Geometry: final body of the model. Coordinates: model frame, mm. Coordinates: 2 decimals unless noted, no trailing zeros. Order: outer loops, then holes, each group sorted by start corner. A loop starts at its lowest first (then second) coordinate and runs counter-clockwise, first axis right, second up. Notation, with made-up numbers: (50, 26.5) - (59, 26.5) arc R8 ccw to (59, 32.5) - close; hole circle Ø1 at (26, 79.25). An arc over 180 degrees is marked (long way). Use a Markdown table: item, result. Add a question column.
```python
from build123d import *

# Parameters (mm, degrees)
F0_W     = 276
F0_H     = 126
F1_DEPTH = 12
F2_R     = 5
F4_W     = 400
F4_H     = 300
F5_DEPTH = 10
F6_R     = 5


with BuildPart() as f1:
    # F0 (on Top) → F1 (new body)
    with BuildSketch(Plane.XY):
        Rectangle(F0_W, F0_H)
    extrude(amount=F1_DEPTH)

    # F2
    f2_edges = [f1.edges().sort_by_distance(p)[0] for p in [
        (0, -63, 12),
        (-138, 0, 12),
        (138, 0, 12),
        (0, 63, 12),
    ]]
    fillet(f2_edges, radius=F2_R)


with BuildPart() as f5:
    # F4 (on Top) → F5 (new body)
    with BuildSketch(Plane.XY):
        Rectangle(F4_W, F4_H)
    extrude(amount=F5_DEPTH)

    # F6
    f6_edges = [f5.edges().sort_by_distance(p)[0] for p in [
        (0, -150, 10),
        (-200, 0, 10),
        (200, 0, 10),
        (0, 150, 10),
    ]]
    fillet(f6_edges, radius=F6_R)


solid = f5.part
```
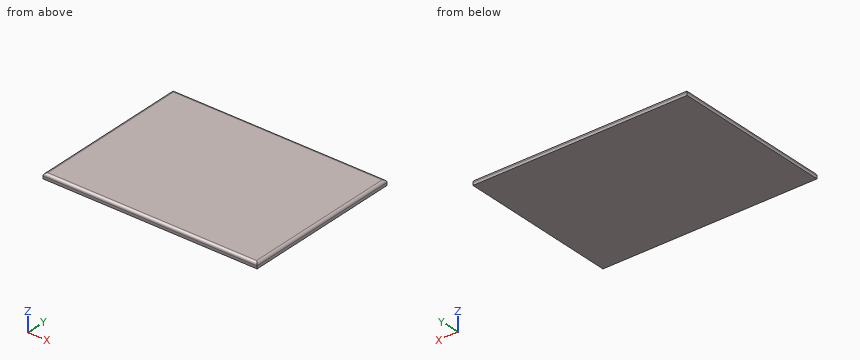
1) First-contact query: pin 1 (5 mm diameter, centred on y = -48, z = 8, fed in from -X). Flat tip, straight axial feed; report the tip coordinate or a pass-through.
2) Line query: line 1 (Y direction, x = 178.5, z = 5.25); line 2 (Y direction, x = -145.5, z = 7); line 3 (X direction, y = 37.5, z = 9). Output: solid intervals per line, ascending. Write a range as from..to.
3) Section query A-A (z = 8.5). Return the cut outline in (x, y), and give its area (3 significant figures).
From the geometry:
| question | item | result |
|---|---|---|
| 1 | pin 1 | stops at x = -199.97 |
| 2 | line 1 | y = -149.99..149.99 |
| 2 | line 2 | y = -149.58..149.58 |
| 2 | line 3 | x = -198..198 |
| 3 | outline | (-198.57, -148.57) - (198.57, -148.57) - (198.57, 148.57) - (-198.57, 148.57) - close |
| 3 | area | 118,000 mm^2 |
